Check sheet for the drawn part. Datum: minimum x, y, z corner. Units: mm. Give positions to 0.01 mm unless a question says otherwise; leave off trailing zeros. Write each loop counter-clockwise with the first axis right and the second up, starting at its lowest first coordinate (ties: lowest second). Pieces come first, ordered by that corner, then holes. Notation, with made-up numbers: (-30, 4.5) -> (24, 4.5) arc R12 ccw to (24, 14.5) -> close; hole circle Ø8 at (59, 7.5). An arc over 180 degrees is marked (long way). Answer as CSV lines item,"result". Start each with the question number.
1) Mould release check, pull along Z, two halves, no side actions. Record for the marked faces 1, 2, 3 and 4: released by +Z, released by -Z, zero draft, split by the parting line, or undercut.
2) Gauge pin test, flat ends, axial feed: pin 1 Ø4.5 at (y, z) = (18.1, 18.1) entering from +X; pin 2 Ø3 at (x, z) = (12.5, 26) entering from +Y; pin 3 Ø2 at (y, z) = (18, 19) entering from -X; pin 4 Ø12 at (y, z) = (18.1, 18.1) entering from +X. Record the tip position at first contact, or that the pin passes through.
3) Sectioned sample at A-A on z = 18.1. Record the cut outline in (x, y).
4) Sectioned sample at C-C on x = 18.25. Record the cut outline in (y, z).
5) Sectioned sample at D-D on y = 7. Record the cut outline in (x, z).
6) Material ranges on L1, parallel to Z at x = 5.25, y = 28.5 (1 decimal); L2, parallel to Z at x = 11.5, y = 3; L3, parallel to Y at x = 14.25, z = 23 (1 decimal), recorded low to high.
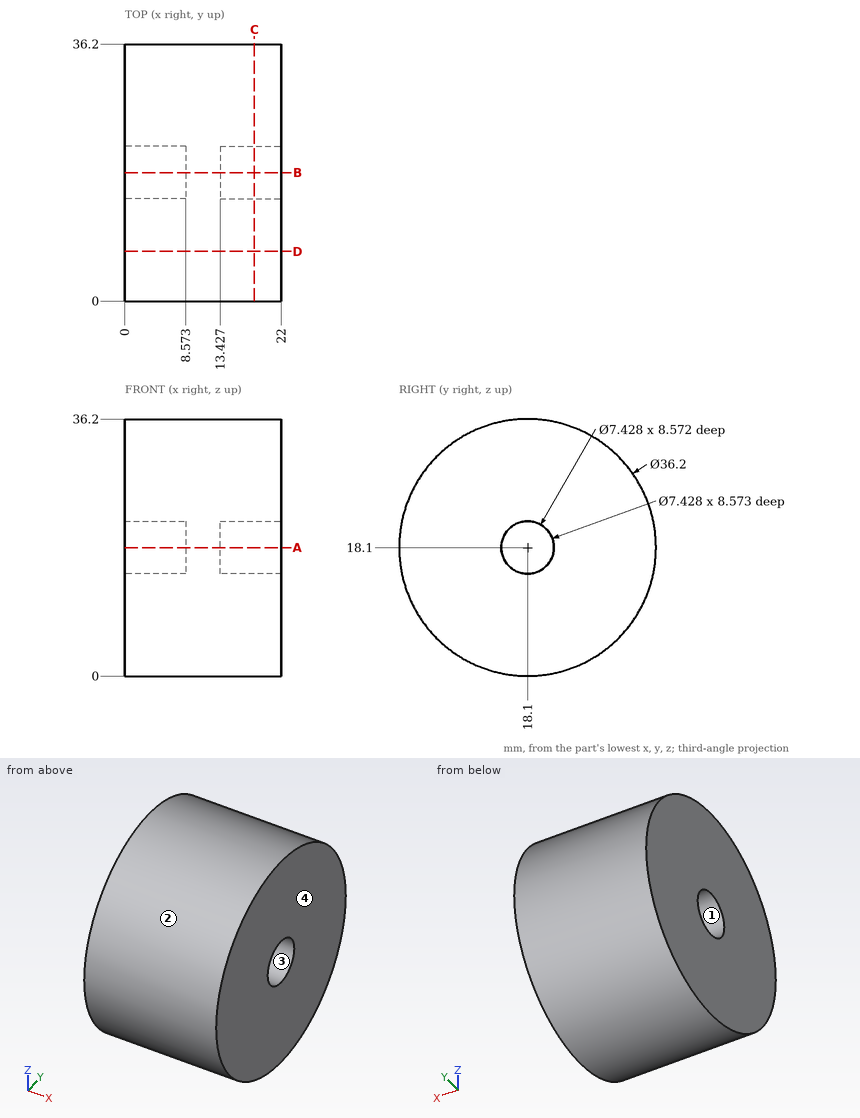
Ans:
1,face 1,"undercut"
1,face 2,"split by the parting line"
1,face 3,"undercut"
1,face 4,"zero draft"
2,pin 1,"stops at x = 13.43"
2,pin 2,"stops at y = 35.03"
2,pin 3,"stops at x = 8.57"
2,pin 4,"stops at x = 22"
3,outline,"(0, 0) -> (22, 0) -> (22, 14.39) -> (13.43, 14.39) -> (13.43, 21.81) -> (22, 21.81) -> (22, 36.2) -> (0, 36.2) -> (0, 21.81) -> (8.57, 21.81) -> (8.57, 14.39) -> (0, 14.39) -> close"
4,outline,"circle Ø36.2 at (18.1, 18.1); hole circle Ø7.43 at (18.1, 18.1)"
5,outline,"(0, 3.8) -> (22, 3.8) -> (22, 32.4) -> (0, 32.4) -> close"
6,L1,"z = 3.3 to 32.9"
6,L2,"z = 8.12 to 28.08"
6,L3,"y = 0.7 to 35.5"
